Read the model definition and answer for the solid it produces. Units are mm, in the model's axes. A direction names the side the tool comes from. Coordinates: 2 decimals unless noted, no trailing zeros. Loops run counter-clockwise (first coordinate to the right, second up) from the corner with the lowest first, then second, coordinate; pieces in that order, holes last. Notation, with made-up numbers: M -22,33.25 L 27,33.25 A32 ccw 27,68.25 Z; hole C 29.5,-7.75 d10. An arc over 180 degrees is marked long. Use one line per item in the form item = value. Start each with the question number.
1. A tool of negligible diameter and unlimited length cuts with its end or side. For faces 4 (the cylindrical face through (59.99, 6.92, -17.36)), 5 (the cylindrical face through (60.07, 196.59, -83.27)), 6 (the flat face through (-86, -36, -68.058)), from which of +Z, -Z, +X, -X, +Y, -Y can it reach the whole face along a straight path? Write none if from no direction.
2. The part is cut by section D-D (x = 107.5). Give the vertices of the cut face in (y, z), plus the area to 3 significant figures.
3. For a pull along Y with two mould halves and no side action, classify faces 1 (the cylindrical face through (-87.86, -13.69, -33.55)), 2 (the flat face through (-42, 3, -98.058)), 3 (the flat face through (0, -62.789, -17)) as released by +Y, released by -Y, zero draft, split by the parting line, or undercut.
4. The part is cut by section A-A (x = 0). Give the vertices of the cut face in (y, z), plus the area to 3 significant figures.
5. Flat-ended cylindrical pins translate along their axes: pin 1 (4 mm diameter, centred on y = -79, z = -0.5, fed in from +X); pin 2 (8.5 mm diameter, centred on y = 71.5, z = -38.5, fed in from +X); pin 3 (1 mm diameter, centred on x = 1, z = -6, fed in from +Y). Find the tip coordinate at first contact, or state that the pin passes through.
6. Find the intervals of material crossed by probe 1 along Z at (x, y) = (176.5, 20.5); probe 2 along Z at (x, y) = (209, -36); probe 3 along Y at (x, z) = (-17.5, -76.5), in increasing order. Write a range as [from, to].
7. The part is cut by section C-C (y = -180.5). Give the vertices of the cut face in (x, z), plus the area to 3 significant figures.
8. The part is cut by section B-B (z = 11). Give the vertices of the cut face in (x, y).
from build123d import *

# Parameters (mm, degrees)
CUT_EXTRUDE1_DEPTH = 100
CIRPATTERN1_COUNT  = 2


with BuildPart() as part:
    # Sketch2 → Revolve1 (revolve)
    with BuildSketch(Plane(origin=(0, 0, 0), x_dir=(0, 0, -1), z_dir=(1, 0, 0))):
        Polygon((-31.942129743, 65.824496016), (-31.942129743, 255.824496016), (-1.942129743, 255.824496016), (-1.942129743, 95.824496016), (68.057870257, 95.824496016), (68.057870257, 205.824496016), (98.057870257, 205.824496016), (98.057870257, 35.824496016), (68.057870257, 35.824496016), (68.057870257, 65.824496016), align=None)
    revolve(axis=Axis((0, 5.824496016, 0), (0, 0, -1)))

    # Sketch3 → Cut-Extrude1 (cut)
    with BuildSketch(Plane.XY.offset(31.942129743)):
        with BuildLine():
            Line((16, 63.651825195), (16, 74.437748913))
            Line((16, 74.437748913), (-16, 74.437748913))
            Line((-16, 74.437748913), (-16, 63.651825195))
            ThreePointArc((-16, 63.651825195), (0, 65.824496016), (16, 63.651825195))
        make_face()
    cut_extrude1 = extrude(amount=-CUT_EXTRUDE1_DEPTH, mode=Mode.SUBTRACT)

    # CirPattern1: Cut-Extrude1 ×2 about axis
    cirpattern1_axis = Axis((0, 5.824496016, 0), (0, 0, 1))
    for i in range(1, CIRPATTERN1_COUNT):
        add(cut_extrude1.rotate(cirpattern1_axis, i * 360 / CIRPATTERN1_COUNT), mode=Mode.SUBTRACT)


solid = part.part
Computed values:
q1.face_4 = +Z
q1.face_5 = -Z
q1.face_6 = none
q2.outline = M -219.88,1.94 L 231.53,1.94 L 231.53,31.94 L -219.88,31.94 Z; M -162.83,-98.06 L 174.48,-98.06 L 174.48,-68.06 L -162.83,-68.06 Z
q2.area = 23,700 mm²
q3.face_1 = split by the parting line
q3.face_2 = zero draft
q3.face_3 = undercut
q4.outline = M -244.18,1.94 L -84.18,1.94 L -84.18,-68.06 L -194.18,-68.06 L -194.18,-98.06 L -24.18,-98.06 L -24.18,-68.06 L -62.79,-68.06 L -62.79,31.94 L -244.18,31.94 Z; M 35.82,-98.06 L 205.82,-98.06 L 205.82,-68.06 L 95.82,-68.06 L 95.82,1.94 L 255.82,1.94 L 255.82,31.94 L 74.44,31.94 L 74.44,-68.06 L 35.82,-68.06 Z
q4.area = 24,100 mm²
q5.pin_1 = 35.22
q5.pin_2 = 65.78
q5.pin_3 = 95.82
q6.probe_1 = [-98.06, -68.06], [1.94, 31.94]
q6.probe_2 = [1.94, 31.94]
q6.probe_3 = [-193.41, -18.54], [30.19, 205.06]
q7.outline = M -166.68,1.94 L 166.68,1.94 L 166.68,31.94 L -166.68,31.94 Z; M -72.69,-98.06 L 72.69,-98.06 L 72.69,-68.06 L -72.69,-68.06 Z
q7.area = 14,400 mm²
q8.outline = C 0,5.82 d500; hole M -16,-62.79 L 16,-62.79 L 16,-52 A60 ccw 16,63.65 L 16,74.44 L -16,74.44 L -16,63.65 A60 ccw -16,-52 Z
